Could you check a few things on this model? Use its own coordinates, in mm. Give positions to 0.01 mm unless a question says otherwise; leave off trailing zeros. Order: outer loops, then holes, each group sorted by start corner. A loop starts at its lowest first (then second) coordinate and runs counter-clockwise, first axis right, second up. Notation, with made-up numbers: M 62.5,71.25 L 102.5,71.25 A34 cw 102.5,107.25 Z; hole C 71.25,57 d9. An arc over 180 degrees is marked long. Return JSON: item names as keys, results as strings. Group by question number.
```python
from build123d import *

# Parameters (mm, degrees)
BOSS_EXTRUDE1_DEPTH = 3


with BuildPart() as part:
    # Sketch1 → Boss-Extrude1 (new body)
    with BuildSketch(Plane(origin=(299.875, 0, 0), x_dir=(0, 0, -1), z_dir=(1, 0, 0))):
        Polygon((254.342966202, 46.438825445), (257.342966202, 46.438825445), (257.342966202, 70.005768865), (261.120760322, 71.404391483), (261.478925383, 63.707591635), (264.650493907, 63.855165721), (264.292328864, 71.551965185), (342.771929635, 71.321990196), (343.128897762, 63.650911904), (346.300465699, 63.798498596), (345.943497573, 71.469576862), (353, 70.477223834), (353, 46.438825445), (356, 46.438825445), (356, 70.477223834), (412.547538785, 65.600801419), (411.981466053, 57.979089008), (415.147745162, 57.743926072), (415.71381799, 65.36563978), (420, 64.4233549), (420, 46.438825445), (423, 46.438825445), (423, 64.4233549), (570, 43.443621916), (570, 31.443621916), (573, 31.443621916), (573, 43.443621916), (583, 43.443621916), (583, 16.438825445), (244.342966202, 16.438825445), (244.342966202, 70.005768865), (254.342966202, 70.005768865), align=None)
    extrude(amount=-BOSS_EXTRUDE1_DEPTH)


solid = part.part
```
1. For pin 1 (0.9 mm diameter, centred on x = 299, z = -421.5, fed in from +Y); pin 2 (0.9 mm diameter, centred on x = 298, z = -572, fed in from +Y), each with a flat end and sliding along its axis, tell me the tip position at first contact or that it passes through.
2. Imagine slicing it at C-C, the plane z = -459. Please give me the cut outline in (x, y) (3 decimals), plus the area to 3 significant figures.
3. Imagine slicing it at B-B, the plane y = 51. Please give me the cut outline in (x, z) (3 decimals), plus the area to 3 significant figures.
4. I need wall thicknesses on L1, parallel to Z at x = 297.15, y = 37; L2, parallel to Y at x = 298.95, z = -262.5; L3, parallel to Y at x = 297.05, z = -310. Which ranges of each line are inside material? Lowest first, please. Write a range as from..to.
5. Imagine slicing it at D-D, the plane z = -524. Please give me the cut outline in (x, y) (3 decimals), plus the area to 3 significant figures.
Values:
{
 "1": {"pin 1": "stops at y = 46.44", "pin 2": "stops at y = 31.44"},
 "2": {"outline": "M 296.875,16.439 L 299.875,16.439 L 299.875,59.285 L 296.875,59.285 Z", "area": "129 mm²"},
 "3": {"outline": "M 296.875,-517.054 L 299.875,-517.054 L 299.875,-423 L 296.875,-423 Z; M 296.875,-420 L 299.875,-420 L 299.875,-356 L 296.875,-356 Z; M 296.875,-353 L 299.875,-353 L 299.875,-257.343 L 296.875,-257.343 Z; M 296.875,-254.343 L 299.875,-254.343 L 299.875,-244.343 L 296.875,-244.343 Z", "area": "791 mm²"},
 "4": {"L1": "z = -583..-573, -570..-244.34", "L2": "y = 16.44..63.76", "L3": "y = 16.44..71.42"},
 "5": {"outline": "M 296.875,16.439 L 299.875,16.439 L 299.875,50.009 L 296.875,50.009 Z", "area": "101 mm²"}
}
